Drawing for the job (mm, zero at the part's lowest x, y, z). Give positions to 0.01 mm unless a question says otherwise; leave off trailing zeros. Order: outer loops, then holes, each group sorted by start corner. A loop starts at its lowest first (then second) coordinate and runs counter-clockwise, first axis right, second up. Notation, with made-up numbers: (27, 66.25) - (71, 66.25) arc R25 cw to (71, 96.25) - close; hole circle Ø8 at (81, 30). An arc over 180 degrees is marked (long way). Use a Markdown table: item, result.
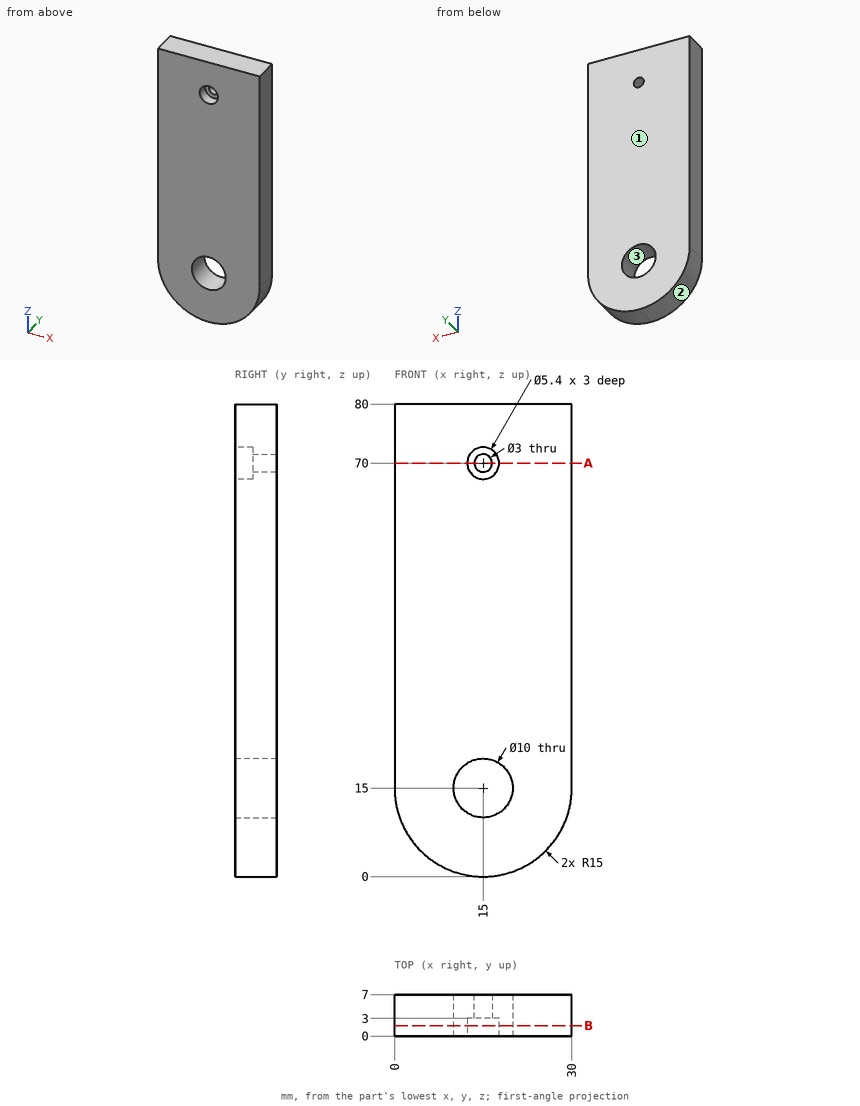
1) Wall check: line 1 (Z direction, x = 15, y = 2.25); line 2 (X direction, y = 3.25, z = 15); line 3 (X direction, y = 4.5, z = 70). Give the ranges that are in metal, low to high. Write a range as from..to.
Computed:
| item | result |
|---|---|
| line 1 | z = 0..10, 20..67.3, 72.7..80 |
| line 2 | x = 0..10, 20..30 |
| line 3 | x = 0..13.5, 16.5..30 |
2) Slice it at A-A (z = 70). Write the cut outline in (x, y).
Computed:
| item | result |
|---|---|
| outline | (0, 0) - (12.3, 0) - (12.3, 3) - (13.5, 3) - (13.5, 7) - (0, 7) - close; (16.5, 3) - (17.7, 3) - (17.7, 0) - (30, 0) - (30, 7) - (16.5, 7) - close |
3) Pin check, flat tips, straight feed: P1, Ø1.8, axis at x = 15, z = 70, coming from the +Y side; P2, Ø1.5, axis at x = 20, y = 4, coming from the -Z side; P3, Ø2.5, axis at x = 14.5, z = 71, coming from the -Y side. Stop position of each tip, or through.
Computed:
| item | result |
|---|---|
| P1 | passes through |
| P2 | stops at z = 0.61 |
| P3 | stops at y = 3 |
4) Slice it at B-B (y = 1.75). State how many separate pieces and enclosed holes the cut face has, and give its area (3 significant figures).
Computed:
| item | result |
|---|---|
| separate pieces | 1 |
| enclosed holes | 2 |
| area | 2,200 mm² |
5) Two-plate mould, pull along X, no slides. Class the marked faces 1, 2 and 3: +X half, -X half, draft (parallel to the pull), parting line (faces both ways), or undercut.
Computed:
| item | result |
|---|---|
| face 1 | draft |
| face 2 | -X half |
| face 3 | undercut |
